from build123d import *

# Parameters (mm, degrees)
BOSS_EXTRUDE1_DEPTH   = 3
CUT_EXTRUDE2_DEPTH    = 1.3
SKETCH4_R             = 20
CUT_EXTRUDE3_DEPTH    = 0.2
F_4_0MM_DOWEL_HOLE1_D = 4
SKETCH8_R             = 2
CUT_EXTRUDE4_DEPTH    = 19


with BuildPart() as part:
    # Sketch1 → Boss-Extrude1 (new body)
    with BuildSketch(Plane(origin=(0, 0, 0), x_dir=(1, 0, 0), z_dir=(0, 1, 0))):
        with BuildLine():
            Line((55.380194412, 68.388844608), (0, 68.388844608))
            Line((0, 68.388844608), (-55.380194412, 68.388844608))
            ThreePointArc((-55.380194412, 68.388844608), (-37.884976519, -79.427505023), (88, 0))
            ThreePointArc((88, 0), (79.427505023, 37.884976519), (55.380194412, 68.388844608))
        make_face()
    extrude(amount=BOSS_EXTRUDE1_DEPTH)

    # Sketch3 → Cut-Extrude2 (cut)
    with BuildSketch(Plane(origin=(0, 3, 0), x_dir=(1, 0, 0), z_dir=(0, 1, 0))):
        Polygon((28, -31.1), (0, -31.1), (-28, -31.1), (-28, 68.388844608), (-31, 68.388844608), (-31, -34.1), (31, -34.1), (31, 68.388844608), (28, 68.388844608), align=None)
    extrude(amount=-CUT_EXTRUDE2_DEPTH, mode=Mode.SUBTRACT)

    # Sketch4 → Cut-Extrude3 (cut)
    with BuildSketch(Plane(origin=(0, 3, 0), x_dir=(1, 0, 0), z_dir=(0, 1, 0))):
        with Locations(Location((35, -54.772, 0), (0, 0, 270))):
            Circle(SKETCH4_R)
        with Locations(Location((-35, -54.472, 0), (0, 0, 270))):
            Circle(SKETCH4_R)
        with Locations(Location((54.772, 35, 0), (0, 0, 270))):
            Circle(SKETCH4_R)
        with Locations(Location((-54.772, 35, 0), (0, 0, 270))):
            Circle(SKETCH4_R)
    extrude(amount=-CUT_EXTRUDE3_DEPTH, mode=Mode.SUBTRACT)

    # Ø4.0mm Dowel Hole1 (through all)
    with Locations(Plane(origin=(-51.423008775, 3, -61.28355545), x_dir=(0, 0, 1), z_dir=(0, 1, 0))):
        with Locations((0, 0), (0, 102.84601755), (140.068175691, 65.314862988), (140.068175691, 37.531154562)):
            Hole(F_4_0MM_DOWEL_HOLE1_D / 2)

    # Sketch8 → Cut-Extrude4 (cut)
    with BuildSketch(Plane(origin=(0, 3, 0), x_dir=(1, 0, 0), z_dir=(0, 1, 0))):
        with Locations(Location((-80, -11, 0), (0, 0, 270))):
            Circle(SKETCH8_R)
        with Locations(Location((80, -11, 0), (0, 0, 270))):
            Circle(SKETCH8_R)
    extrude(amount=-CUT_EXTRUDE4_DEPTH, mode=Mode.SUBTRACT)


solid = part.part
Verification items for the finished model (mm, model axes). A direction names the side the tool comes from. Coordinates: 2 decimals unless noted, no trailing zeros. Order: outer loops, then holes, each group sorted by start corner. A loop starts at its lowest first (then second) coordinate and runs counter-clockwise, first axis right, second up. Notation, with made-up numbers: (-23.75, -13.75) -> (-17.75, -13.75) arc R18 ccw to (-17.75, -0.75) -> close; hole circle Ø1 at (24, 48.5). An arc over 180 degrees is marked (long way). Use CSV: the item, a comma, the result in double quotes. Start each with the question number.
Q1. Section check B-B, the plane y = 1.2. Record the cut outline in (x, z), and give its area (3 significant figures).
Q2. Tool access check on faces 3 (the cylindrical face through (14.493, 1.479, 76.877)), 4 (the flat face through (35, 2.8, 54)). Record the directions out of +Z, -Z, +X, -X, +Y, -Y that give a thin tool (end or side, any length) a straight path to the whole face; none if there is none.
Q3. Thickness scan on line 1 along X through (y, z) = (2.7, 30); line 2 along Y through (x, z) = (-45, -18); line 3 along X through (y, z) = (1.05, 11). Record the ranges inside material, lowest first.
Q4. Depth check by flat-ended pin: P1, Ø1.4, axis at y = 2, z = 3.5, coming from the +X side; P2, Ø1, axis at y = 2, z = -28.5, coming from the -X side; P3, Ø24, axis at x = -35, z = 54.472, coming from the +Y side. Enter the tip coordinate at first touch or a pass-through.
Q5. Section check D-D, the plane z = -11. Record the cut outline in (x, y).
Q6. Draft check along Z on faces 1 (the cylindrical face through (-49.44, 1.48, -61.02)), 2 (the flat face through (-1, 0, 9)). Enter one of: +Z half, -Z half, draft (parallel to the pull), parting line (faces both ways), or undercut.
Q7. Section check C-C, the plane x = 80. Record the cut outline in (y, z).
Q8. Section check A-A, the plane z = 11. Record the cut outline in (x, y).
Returned:
1,outline,"(-55.38, -68.39) -> (55.38, -68.39) arc R88 ccw (long way) to start; hole circle Ø4 at (-80, 11); hole circle Ø4 at (-51.42, -61.28); hole circle Ø4 at (-13.89, 78.78); hole circle Ø4 at (13.89, 78.78); hole circle Ø4 at (51.42, -61.28); hole circle Ø4 at (80, 11)"
1,area,"22,800 mm^2"
2,face 3,"+Y, -Y"
2,face 4,"+Y"
3,line 1,"x = -82.73 to -31, -28 to 28, 31 to 82.73"
3,line 2,"y = 0 to 2.8"
3,line 3,"x = -87.31 to -82, -78 to 78, 82 to 87.31"
4,P1,"stops at x = 87.96"
4,P2,"stops at x = -83.43"
4,P3,"stops at y = 2.8"
5,outline,"(-87.31, 0) -> (87.31, 0) -> (87.31, 3) -> (31, 3) -> (31, 1.7) -> (28, 1.7) -> (28, 3) -> (-28, 3) -> (-28, 1.7) -> (-31, 1.7) -> (-31, 3) -> (-87.31, 3) -> close"
6,face 1,"undercut"
6,face 2,"draft"
7,outline,"(0, -36.66) -> (3, -36.66) -> (3, 9) -> (0, 9) -> close; (0, 13) -> (3, 13) -> (3, 36.66) -> (0, 36.66) -> close"
8,outline,"(-87.31, 0) -> (-82, 0) -> (-82, 3) -> (-87.31, 3) -> close; (-78, 0) -> (78, 0) -> (78, 3) -> (31, 3) -> (31, 1.7) -> (28, 1.7) -> (28, 3) -> (-28, 3) -> (-28, 1.7) -> (-31, 1.7) -> (-31, 3) -> (-78, 3) -> close; (82, 0) -> (87.31, 0) -> (87.31, 3) -> (82, 3) -> close"
